Autodesk Inventor part; units mm, degrees
ref_plane "YZ Plane" through (0, 0, 0) normal (1, 0, 0) x (0, 1, 0)
ref_plane "XZ Plane" through (0, 0, 0) normal (0, 1, 0) x (-1, 0, 0)
ref_plane "XY Plane" through (0, 0, 0) normal (0, 0, 1) x (1, 0, 0)
sketch "Sketch1" plane through (0, 0, 0) normal (0, 0, 1) x (1, 0, 0)
  line L0 (2.6235, 11.5434) -> (28.0235, 11.5434)
  line L1 (28.0235, 11.5434) -> (28.0235, 14.7184)
  line L2 (28.0235, 14.7184) -> (2.6235, 14.7184)
  line L3 (2.6235, 14.7184) -> (2.6235, 11.5434)
  line L4 (28.0235, -8.7766) -> (2.6235, -8.7766)
  line L5 (2.6235, -8.7766) -> (2.6235, -11.9516)
  line L6 (2.6235, -11.9516) -> (28.0235, -11.9516)
  line L7 (28.0235, -11.9516) -> (28.0235, -8.7766)
  line L8 (28.0235, -11.9516) -> (34.3735, -11.9516)
  line L9 (34.3735, -11.9516) -> (34.3735, 14.7184)
  line L10 (34.3735, 14.7184) -> (28.0235, 14.7184)
  line L11 (28.0235, 14.7184) -> (28.0235, -11.9516)
  line L12 (2.6235, -50.4767) -> (53.4235, -50.4767)
  line L13 (53.4235, -50.4767) -> (53.4235, -44.1267)
  line L14 (53.4235, -44.1267) -> (2.6235, -44.1267)
  line L15 (2.6235, -44.1267) -> (2.6235, -50.4767)
  line L16 (53.4235, -50.4767) -> (59.7735, -50.4767)
  line L17 (59.7735, -50.4767) -> (59.7735, 0.3233)
  line L18 (59.7735, 0.3233) -> (53.4235, 0.3233)
  line L19 (53.4235, 0.3233) -> (53.4235, -50.4767)
  line L20 (34.3735, -11.9516) -> (53.4235, -11.9516)
  line L21 (59.7735, 0.3233) -> (34.3735, 14.7184)
  point P0 (0, 0)
  dimension "d22" = 27.94
  dimension "d0" = 25.4
  dimension "d1" = 3.175
  dimension "d2" = 3.175
  dimension "d3" = 20.32
  dimension "d4" = 6.35
  dimension "d5" = 50.8
  dimension "d6" = 6.35
  dimension "d7" = 6.35
  dimension "d8" = 50.8
extrude "Extrusion1" add sketch "Sketch1" along normal blind 38.1
sketch "Sketch2" plane through (59.7735, -50.4767, 0) normal (1, 0, 0) x (0, 0, -1)
  circle A0 centre (-12.7, 25.4) radius 3.175
  line L0 (0, 50.8) -> (-38.1, 50.8)
  line L1 (-38.1, 0) -> (-38.1, 50.8)
  point P0 (0, 50.4767)
  dimension "d11" = 6.35
  dimension "d12" = 25.4
  dimension "d13" = 25.4
extrude "Extrusion2" cut sketch "Sketch2" against normal blind 25.4
sketch "Sketch3" plane through (2.6235, 14.7184, 0) normal (0, 1, 0) x (1, 0, 0)
  circle A0 centre (3.175, -6.35) radius 1.5875
  circle A1 centre (20.775, -6.35) radius 1.5875
  line L0 (31.75, 0) -> (0, 0)
  line L1 (0, 0) -> (0, -38.1)
  point P0 (-2.6235, 0)
  dimension "d16" = 3.175
  dimension "d17" = 3.175
  dimension "d18" = 6.35
  dimension "d19" = 6.35
  dimension "d20" = 17.6
  dimension "d21" = 3.175
extrude "Extrusion3" cut sketch "Sketch3" against normal blind 27.94
fillet "Fillet1" radius 3.175 7 edges at (34.3735, 14.7184, 19.05) (59.7735, 0.3233, 19.05) (59.7735, -50.4767, 19.05) (53.4235, -11.9516, 19.05) (53.4235, -44.1267, 19.05) (2.6235, -50.4767, 19.05) (2.6235, -44.1267, 19.05)
fillet "Fillet2" radius 0.508 6 edges at (2.6235, -8.7766, 19.05) (2.6235, -11.9516, 19.05) (2.6235, 11.5434, 19.05) (2.6235, 14.7184, 19.05) (28.0235, 11.5434, 19.05) (28.0235, -8.7766, 19.05)
sketch "Sketch4" plane through (5.7985, -50.4767, 0) normal (0, -1, 0) x (1, 0, 0)
  circle A0 centre (9.525, 26.67) radius 4.445
  line L0 (-3.175, 38.1) -> (-3.175, 0)
  line L1 (0, 38.1) -> (50.8, 38.1)
  point P0 (-5.7985, 0)
  dimension "d26" = 8.89
  dimension "d28" = 12.7
  dimension "d29" = 11.43
extrude "Extrusion4" cut sketch "Sketch4" against normal blind 101.6
sketch "Sketch5" plane through (50.2485, -11.9516, 0) normal (0, -1, 0) x (1, 0, 0)
  circle A0 centre (-34.925, 26.67) radius 4.445
  circle A1 centre (-34.925, 26.67) radius 6.35
  point P0 (-50.2485, 0)
  dimension "d32" = 12.7
extrude "Extrusion5" cut sketch "Sketch5" against normal blind 5.08
equation "\"d14\" = d12"
properties part number "SwerveBracket"
Check sheet for the modelled part. Datum: model origin and axes. Units: mm. A direction names the side the tool comes from. Give positions to 0.01 mm unless a question says otherwise; leave off trailing zeros. Loops run counter-clockwise (first coordinate to the right, second up) from the corner with the lowest first, then second, coordinate; pieces in that order, holes last. Notation, with made-up numbers: M -25,-18 L -4,-18 A29 cw -4,9 Z; hole C -26,-20 d10. An arc over 180 degrees is marked long. Return JSON: item names as keys, results as strings. Group by question number.
1. Tool access check on faces 5 (the flat face through (28, -44.127, 19)), 6 (the flat face through (59.774, -25, 19)), 7 (the cylindrical face through (7.265, 13.153, 6.958)). Record the directions out of +Z, -Z, +X, -X, +Y, -Y that give a thin tool (end or side, any length) a straight path to the whole face; none if there is none.
2. Mould release check, pull along Y, two halves, no side actions. Record for faces 1 (the flat face through (53.424, -28, 19)), 2 (the cylindrical face through (24.865, -10.342, 6.958)), 3 (the cylindrical face through (3.529, -49.522, 19.317)), 4 (the cylindrical face through (59.354, 0.051, 19.317)): released by +Y, released by -Y, zero draft, split by the parting line, or undercut.
3. Cross-section at D-D on z = 26.67. State how many separate pieces and enclosed holes the cut face has, plus the area to 3 significant figures.
4. Cross-section at C-C on x = 14. Record the boundary of the cut face in (y, z).
5. Cross-section at A-A on x = 47. Record the boundary of the cut face in (y, z), plus the area to 3 significant figures.
6. Go/stop test with flat-tipped pins: pin 1 (1.9 mm diameter, centred on x = 5.8, z = 6.35, fed in from +Y); pin 2 (8 mm diameter, centred on y = -26, z = 8, fed in from -X); pin 3 (1.5 mm diameter, centred on x = 46, z = 32, fed in from +Y). Record where each tip stops, or that it passes through.
7. Thickness scan on L1, parallel to Y at x = 9, z = 20; L2, parallel to X at y = 13, z = 6; L3, parallel to X at y = 13, z = 6.35. Record the ranges inside material, lowest first.
Return value:
{
 "1": {"face 5": "+Z, -Z, -X", "face 6": "+Z, -Z, +X, +Y, -Y", "face 7": "+Y"},
 "2": {"face 1": "undercut", "face 2": "zero draft", "face 3": "released by -Y", "face 4": "released by +Y"},
 "3": {"separate pieces": "4", "enclosed holes": "0", "area": "1,260 mm^2"},
 "4": {"outline": "M -50.48,0 L -44.13,0 L -44.13,22.43 L -50.48,22.43 Z; M -50.48,30.91 L -44.13,30.91 L -44.13,38.1 L -50.48,38.1 Z; M -11.95,0 L -8.78,0 L -8.78,20.46 L -11.95,20.46 Z; M -11.95,32.88 L -8.78,32.88 L -8.78,38.1 L -11.95,38.1 Z; M 11.54,0 L 14.72,0 L 14.72,22.43 L 11.54,22.43 Z; M 11.54,30.91 L 14.72,30.91 L 14.72,38.1 L 11.54,38.1 Z"},
 "5": {"outline": "M -50.48,0 L -44.13,0 L -44.13,38.1 L -50.48,38.1 Z; M -11.95,0 L 7.56,0 L 7.56,38.1 L -11.95,38.1 Z", "area": "985 mm^2"},
 "6": {"pin 1": "y = -44.13", "pin 2": "x = 53.42", "pin 3": "y = 8.55"},
 "7": {"L1": "-50.48 to -44.13, -11.95 to -8.78, 11.54 to 14.72", "L2": "2.62 to 4.25, 7.35 to 21.85, 24.95 to 37.41", "L3": "2.62 to 4.21, 7.39 to 21.81, 24.99 to 37.41"}
}
